Check sheet for the modelled part. Datum: model origin and axes. Units: mm. Face numbers are marked on the shaded views. A direction names the side the tool comes from. Round coordinates to 2 decimals unless told otherwise and drop trailing zeros. Loops run counter-clockwise (first coordinate to the right, second up) from the corner with the lowest first, then second, coordinate; pieces in that order, holes last. Notation, with made-up numbers: (44, 34.25) - (60, 34.25) arc R24 ccw to (60, 72.25) - close; hole circle Ø11 at (-2.75, 1.25). An arc over 180 degrees is marked (long way). Put each result on its own line as item: value. Start each with the question number.
Item 1: Section check A-A, the plane x = 0. Give the number of separate pieces and of enclosed holes in the cut face, and give its area (3 significant figures).
Item 2: Section check C-C, the plane y = -30. Record the cut outline in (x, z), and give its area (3 significant figures).
Item 3: Material ranges on line 1 along Z through (x, y) = (36.3, 0); line 2 along Y through (x, z) = (-4.5, 4.65); line 3 along Y through (x, z) = (-17, 0.45), recorded low to high.
Item 4: Section check D-D, the plane x = 12.5. Record the cut outline in (y, z), and give its area (3 significant figures).
Item 5: Gauge pin test, flat ends, axial feed: pin 1 Ø2 at (x, z) = (0, 2.65) entering from -Y; pin 2 Ø3 at (x, z) = (-3, 4) entering from -Y; pin 3 Ø3 at (y, z) = (-22, 2.5) entering from +X; pin 4 Ø1 at (x, z) = (-18.5, 1.5) entering from -Y. Record the tip position at first contact, or that the pin passes through.
Item 6: Tool access check on the marked faces 3 and 4. Record the directions out of +Z, -Z, +X, -X, +Y, -Y that give a thin tool (end or side, any length) a straight path to the whole face; none if there is none.
Item 7: Draft check along X on the marked faces 1 and 2. Enter one of: pulls with the +X half, pulls with the -X half, needs draft (parallel to the pull), parting line crosses it, or undercut.
from build123d import *

# Parameters (mm, degrees)
BOSS_EXTRUDE1_DEPTH = 5
CUT_EXTRUDE2_START  = -4
SKETCH3_R           = 1.1
CUT_EXTRUDE2_DEPTH  = 5
CIRPATTERN7_COUNT   = 4
SKETCH4_R           = 37.79
BOSS_EXTRUDE2_DEPTH = 5
SKETCH5_R           = 1.1
CUT_EXTRUDE3_DEPTH  = 13.35
CIRPATTERN8_COUNT   = 4


with BuildPart() as part:
    # Sketch1 → Boss-Extrude1 (new body)
    with BuildSketch(Plane.XY):
        with BuildLine():
            Line((-6.1, 25.44), (6.1, 25.44))
            ThreePointArc((6.1, 25.44), (18.498697251, 18.498697251), (25.44, 6.1))
            Line((25.44, 6.1), (25.44, -6.1))
            ThreePointArc((25.44, -6.1), (18.498697251, -18.498697251), (6.1, -25.44))
            Line((6.1, -25.44), (-6.1, -25.44))
            ThreePointArc((-6.1, -25.44), (-18.498697251, -18.498697251), (-25.44, -6.1))
            Line((-25.44, -6.1), (-25.44, 6.1))
            ThreePointArc((-25.44, 6.1), (-18.498697251, 18.498697251), (-6.1, 25.44))
        make_face()
        with BuildLine():
            Line((-6.1, 21.44), (6.1, 21.44))
            ThreePointArc((6.1, 21.44), (15.76203667, 15.76203667), (21.44, 6.1))
            Line((21.44, 6.1), (21.44, -6.1))
            ThreePointArc((21.44, -6.1), (15.76203667, -15.76203667), (6.1, -21.44))
            Line((6.1, -21.44), (-6.1, -21.44))
            ThreePointArc((-6.1, -21.44), (-15.76203667, -15.76203667), (-21.44, -6.1))
            Line((-21.44, -6.1), (-21.44, 6.1))
            ThreePointArc((-21.44, 6.1), (-15.76203667, 15.76203667), (-6.1, 21.44))
        make_face(mode=Mode.SUBTRACT)
    extrude(amount=BOSS_EXTRUDE1_DEPTH)

    # Sketch3 → Cut-Extrude2 (cut)
    with BuildSketch(Plane(origin=(0, 25.44, 0), x_dir=(1, 0, 0), z_dir=(0, 1, 0)).offset(CUT_EXTRUDE2_START)):
        with Locations((0, -2.65)):
            Circle(SKETCH3_R)
    cut_extrude2 = extrude(amount=CUT_EXTRUDE2_DEPTH, mode=Mode.SUBTRACT)

    # CirPattern7: Cut-Extrude2 ×4 about axis
    cirpattern7_axis = Axis((0, 0, 5), (0, 0, -1))
    for i in range(1, CIRPATTERN7_COUNT):
        add(cut_extrude2.rotate(cirpattern7_axis, i * 360 / CIRPATTERN7_COUNT), mode=Mode.SUBTRACT)

    # Sketch4 → Boss-Extrude2 (add)
    with BuildSketch(Plane.XY.offset(5)):
        Circle(SKETCH4_R)
        with BuildLine():
            Line((-25.650884562, 24.236671), (-19.192284627, 17.778071065))
            ThreePointArc((-19.192284627, 17.778071065), (-18.498697251, 18.498697251), (-17.778071065, 19.192284627))
            Line((-17.778071065, 19.192284627), (-24.236671, 25.650884562))
            ThreePointArc((-24.236671, 25.650884562), (0, 35.29), (24.236671, 25.650884562))
            Line((24.236671, 25.650884562), (17.778071065, 19.192284627))
            ThreePointArc((17.778071065, 19.192284627), (18.498697251, 18.498697251), (19.192284627, 17.778071065))
            Line((19.192284627, 17.778071065), (25.650884562, 24.236671))
            ThreePointArc((25.650884562, 24.236671), (35.29, 0), (25.650884562, -24.236671))
            Line((25.650884562, -24.236671), (19.192284627, -17.778071065))
            ThreePointArc((19.192284627, -17.778071065), (18.498697251, -18.498697251), (17.778071065, -19.192284627))
            Line((17.778071065, -19.192284627), (24.236671, -25.650884562))
            ThreePointArc((24.236671, -25.650884562), (0, -35.29), (-24.236671, -25.650884562))
            Line((-24.236671, -25.650884562), (-17.778071065, -19.192284627))
            ThreePointArc((-17.778071065, -19.192284627), (-18.498697251, -18.498697251), (-19.192284627, -17.778071065))
            Line((-19.192284627, -17.778071065), (-25.650884562, -24.236671))
            ThreePointArc((-25.650884562, -24.236671), (-35.29, 0), (-25.650884562, 24.236671))
        make_face(mode=Mode.SUBTRACT)
    extrude(amount=-BOSS_EXTRUDE2_DEPTH)

    # Sketch5 → Cut-Extrude3 (cut, through all)
    with BuildSketch(Plane.ZY.offset(25.44)):
        with Locations((2.65, 0)):
            Circle(SKETCH5_R)
    cut_extrude3 = extrude(amount=CUT_EXTRUDE3_DEPTH, mode=Mode.SUBTRACT)

    # CirPattern8: Cut-Extrude3 ×4 about axis
    cirpattern8_axis = Axis((0, 0, -106.886261044), (0, 0, 1))
    for i in range(1, CIRPATTERN8_COUNT):
        add(cut_extrude3.rotate(cirpattern8_axis, i * 360 / CIRPATTERN8_COUNT), mode=Mode.SUBTRACT)


solid = part.part
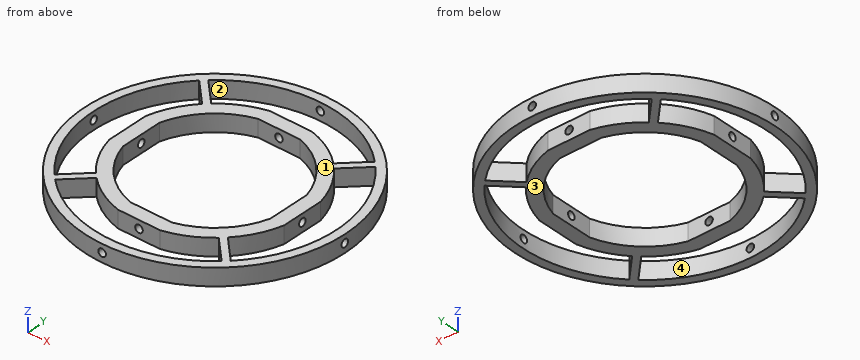
Check result:
1. separate pieces: 8
1. enclosed holes: 0
1. area: 36.4 mm²
2. outline: (-22.98, 0) - (-18.58, 0) - (-18.58, 5) - (-22.98, 5) - close; (18.58, 0) - (22.98, 0) - (22.98, 5) - (18.58, 5) - close
2. area: 44.0 mm²
3. line 1: 0 to 1.55, 3.75 to 5
3. line 2: -37.52 to -35, -25.44 to -21.44, 21.44 to 25.44, 35 to 37.52
3. line 3: -33.75 to -30.93, -19.88 to -14.42, 14.42 to 19.88, 30.93 to 33.75
4. outline: (-35.66, 0) - (-33, 0) - (-33, 5) - (-35.66, 5) - close; (-22.98, 0) - (-18.46, 0) - (-18.46, 5) - (-22.98, 5) - close; (18.46, 0) - (22.98, 0) - (22.98, 5) - (18.46, 5) - close; (33, 0) - (35.66, 0) - (35.66, 5) - (33, 5) - close
4. area: 71.9 mm²
5. pin 1: through
5. pin 2: y = -37.76
5. pin 3: x = 31.75
5. pin 4: y = -33.23
6. face 3: -Z, +X, -X, +Y, -Y
6. face 4: +Z, -Z
7. face 1: needs draft
7. face 2: undercut
